```python
from build123d import *

# Parameters (mm, degrees)
F0_W      = 15.748
F0_H      = 15.748
F1_DEPTH  = 9.5758
F2_R      = 2.4511
F4_DEPTH  = 1.905
F3_R      = 2.4511
F5_DEPTH  = 1.905
F6_R      = 2.4511
F7_DEPTH  = 1.905
F8_W      = 13.2842
F8_H      = 14.089584
F9_DEPTH  = 7.62
F10_R     = 3.2385
F11_DEPTH = 7.62


with BuildPart() as f1:
    # F0 (on Top) → F1 (new body)
    with BuildSketch(Plane.XY):
        Rectangle(F0_W, F0_H)
    extrude(amount=F1_DEPTH)

    # F2 (on face) → F4 (join)
    with BuildSketch(Plane.XY.offset(9.5758)):
        with Locations((-3.7719, 3.7719)):
            Circle(F2_R)
    extrude(amount=F4_DEPTH)

    # F3 (on face) → F5 (join)
    with BuildSketch(Plane.XY.offset(9.5758)):
        with Locations((-3.7719, -3.7719)):
            Circle(F3_R)
    extrude(amount=F5_DEPTH)

    # F6 (on face) → F7 (join)
    with BuildSketch(Plane.XY.offset(9.5758)):
        with Locations((3.7719, 3.7719)):
            Circle(F6_R)
        with Locations((3.7719, -3.7719)):
            Circle(F6_R)
    extrude(amount=F7_DEPTH)

    # F8 (on face) → F9 (cut)
    with BuildSketch(Plane(origin=(0, 0, 0), x_dir=(1, 0, 0), z_dir=(0, 0, -1))):
        Rectangle(F8_W, F8_H)
    extrude(amount=-F9_DEPTH, mode=Mode.SUBTRACT)

    # F10 (on face) → F11 (join)
    with BuildSketch(Plane(origin=(0, 0, 7.62), x_dir=(1, 0, 0), z_dir=(0, 0, -1))):
        Circle(F10_R)
    extrude(amount=F11_DEPTH)


solid = f1.part
```
Input: part model. Units: mm. Frame: model coordinates. A direction names the side the tool comes from. Coordinates: 2 decimals unless noted, no trailing zeros. Loops run counter-clockwise (first coordinate to the right, second up) from the corner with the lowest first, then second, coordinate; pieces in that order, holes last. Notation, with made-up numbers: (54, -22) - (61, -22) arc R32 ccw to (61, 15) - close; hole circle Ø3 at (56, 14). An arc over 180 degrees is marked (long way). Answer in a Markdown table with one row per item.
(1) Cut plane A-A on z = 5. Output: boundary loops of the cut face in (x, y), plus the area to 3 significant figures.
Model answer:
| item | result |
|---|---|
| outline | (-7.87, -7.87) - (7.87, -7.87) - (7.87, 7.87) - (-7.87, 7.87) - close; circle Ø6.48 at (0, 0); hole (-6.64, -7.04) - (6.64, -7.04) - (6.64, 7.04) - (-6.64, 7.04) - close |
| area | 93.8 mm² |
(2) Set-up query: faces 4 (the face through (0, -7.045, 4)), 5 (the face through (7.874, 0, 5)), 6 (the face through (0, 0, 9.576)). Return all of +Z, -Z, +X, -X, +Y, -Y with unobstructed straight access to the full face (end or side cutting, diameter ignored); none if empty.
Model answer:
| item | result |
|---|---|
| face 4 | -Z |
| face 5 | +Z, -Z, +X, +Y, -Y |
| face 6 | +Z |
(3) Cut plane B-B on x = 0. Output: boundary loops of the cut face in (y, z).
Model answer:
| item | result |
|---|---|
| outline | (-7.87, 0) - (-7.04, 0) - (-7.04, 7.62) - (-3.24, 7.62) - (-3.24, 0) - (3.24, 0) - (3.24, 7.62) - (7.04, 7.62) - (7.04, 0) - (7.87, 0) - (7.87, 9.58) - (-7.87, 9.58) - close |
(4) Cut plane C-C on y = 0. Output: boundary loops of the cut face in (x, z).
Model answer:
| item | result |
|---|---|
| outline | (-7.87, 0) - (-6.64, 0) - (-6.64, 7.62) - (-3.24, 7.62) - (-3.24, 0) - (3.24, 0) - (3.24, 7.62) - (6.64, 7.62) - (6.64, 0) - (7.87, 0) - (7.87, 9.58) - (-7.87, 9.58) - close |
(5) Material intervals for L1, parallel to Y at x = 6.25, z = 1; L2, parallel to Y at x = -3.75, z = 10; L3, parallel to X at y = 3.5, z = 2.25, sorted ascending. Write a range as from..to.
Model answer:
| item | result |
|---|---|
| L1 | y = -7.87..-7.04, 7.04..7.87 |
| L2 | y = -6.22..-1.32, 1.32..6.22 |
| L3 | x = -7.87..-6.64, 6.64..7.87 |
(6) Cut plane D-D on x = -1.75. Output: boundary loops of the cut face in (y, z).
Model answer:
| item | result |
|---|---|
| outline | (-7.87, 0) - (-7.04, 0) - (-7.04, 7.62) - (-2.72, 7.62) - (-2.72, 0) - (2.72, 0) - (2.72, 7.62) - (7.04, 7.62) - (7.04, 0) - (7.87, 0) - (7.87, 9.58) - (5.16, 9.58) - (5.16, 11.48) - (2.39, 11.48) - (2.39, 9.58) - (-2.39, 9.58) - (-2.39, 11.48) - (-5.16, 11.48) - (-5.16, 9.58) - (-7.87, 9.58) - close |
(7) Mould query, pull axis Y, two halves, no side actions, for faces 1 (the face through (-0.7, 3.16, 3.86)), 2 (the face through (0, -7.874, 5)), 3 (the face through (-4, 4, 11.481)). Classes: pulls with the +Y half, pulls with the -Y half, needs draft (parallel to the pull), parting line crosses it, or undercut.
Model answer:
| item | result |
|---|---|
| face 1 | undercut |
| face 2 | pulls with the -Y half |
| face 3 | needs draft |
